```python
from build123d import *

# Parameters (mm, degrees)
F0_R     = 11.2
F0_R_2   = 13.2
F1_DEPTH = 7


with BuildPart() as f1:
    # F0 (on Top) → F1 (new body)
    with BuildSketch(Plane.XY):
        with BuildLine():
            ThreePointArc((6.699736, 20.60143), (11.46029, 25.424858), (13.2, 31.9748))
            ThreePointArc((13.2, 31.9748), (13.048167, 33.971132), (12.59616, 35.921539))
            ThreePointArc((12.59616, 35.921539), (11.664432, 38.15388), (10.34098, 40.17871))
            ThreePointArc((10.34098, 40.17871), (-6.83944, 43.26471), (-12.059859, 26.608256))
            ThreePointArc((-12.059859, 26.608256), (-10.553777, 24.046509), (-8.512807, 21.886583))
            ThreePointArc((-8.512807, 21.886583), (-6.711654, 20.60846), (-4.722613, 19.64853))
            ThreePointArc((-4.722613, 19.64853), (-0.715754, 18.79422), (3.360055, 19.209612))
            ThreePointArc((3.360055, 19.209612), (5.077808, 19.790553), (6.699736, 20.60143))
        make_face()
        with Locations((0, 31.9748)):
            Circle(F0_R, mode=Mode.SUBTRACT)
        with BuildLine():
            ThreePointArc((10.34098, 40.17871), (11.664432, 38.15388), (12.59616, 35.921539))
            ThreePointArc((12.59616, 35.921539), (18.781531, 26.896904), (19.593705, 15.986211))
            ThreePointArc((19.593705, 15.986211), (21.142377, 14.729254), (22.578902, 13.345517))
            ThreePointArc((22.578902, 13.345517), (21.814507, 29.204192), (10.34098, 40.17871))
        make_face()
        with BuildLine():
            ThreePointArc((19.593705, 15.986211), (13.490319, 19.253765), (6.699736, 20.60143))
            ThreePointArc((6.699736, 20.60143), (5.077808, 19.790553), (3.360055, 19.209612))
            ThreePointArc((3.360055, 19.209612), (17.479874, 11.47432), (23.21074, -3.570985))
            ThreePointArc((23.21074, -3.570985), (26.101776, -2.883416), (29.073356, -2.859984))
            ThreePointArc((29.073356, -2.859984), (27.386598, 5.868135), (22.578902, 13.345517))
            ThreePointArc((22.578902, 13.345517), (21.142377, 14.729254), (19.593705, 15.986211))
        make_face()
        with BuildLine():
            ThreePointArc((-8.512807, 21.886583), (-10.553777, 24.046509), (-12.059859, 26.608256))
            ThreePointArc((-12.059859, 26.608256), (-18.775253, 20.783423), (-22.847008, 12.881144))
            ThreePointArc((-22.847008, 12.881144), (-23.327096, 10.945209), (-23.641317, 8.97554))
            ThreePointArc((-23.641317, 8.97554), (-23.419409, 2.056076), (-21.191229, -4.498574))
            ThreePointArc((-21.191229, -4.498574), (-19.678026, -5.497766), (-18.316039, -6.694913))
            ThreePointArc((-18.316039, -6.694913), (-18.67699, 9.400855), (-8.512807, 21.886583))
        make_face()
        with BuildLine():
            ThreePointArc((23.21074, -3.570985), (21.203277, -4.491767), (19.377433, -5.734362))
            ThreePointArc((19.377433, -5.734362), (16.634148, -8.777249), (14.955984, -12.514699))
            ThreePointArc((14.955984, -12.514699), (14.600218, -14.292788), (14.491494, -16.102856))
            ThreePointArc((14.491494, -16.102856), (17.425303, -24.285333), (24.810885, -28.869364))
            ThreePointArc((24.810885, -28.869364), (27.210013, -29.178634), (29.625294, -29.044906))
            ThreePointArc((29.625294, -29.044906), (37.685308, -24.610253), (40.890989, -15.9874))
            ThreePointArc((40.890989, -15.9874), (37.501372, -7.155844), (29.073356, -2.859984))
            ThreePointArc((29.073356, -2.859984), (26.101776, -2.883416), (23.21074, -3.570985))
        make_face()
        with Locations((27.690989, -15.9874)):
            Circle(F0_R, mode=Mode.SUBTRACT)
        with BuildLine():
            ThreePointArc((-23.641317, 8.97554), (-23.327096, 10.945209), (-22.847008, 12.881144))
            ThreePointArc((-22.847008, 12.881144), (-36.198826, 4.289821), (-39.966273, -11.133804))
            ThreePointArc((-39.966273, -11.133804), (-38.874445, -8.975245), (-37.407045, -7.052174))
            ThreePointArc((-37.407045, -7.052174), (-32.684167, 2.816831), (-23.641317, 8.97554))
        make_face()
        with BuildLine():
            ThreePointArc((-14.65482, -13.914168), (-15.918395, -10.016971), (-18.316039, -6.694913))
            ThreePointArc((-18.316039, -6.694913), (-19.678026, -5.497766), (-21.191229, -4.498574))
            ThreePointArc((-21.191229, -4.498574), (-29.744367, -2.948089), (-37.407045, -7.052174))
            ThreePointArc((-37.407045, -7.052174), (-38.874445, -8.975245), (-39.966273, -11.133804))
            ThreePointArc((-39.966273, -11.133804), (-34.048618, -27.555484), (-17.013496, -23.748273))
            ThreePointArc((-17.013496, -23.748273), (-15.547999, -21.163093), (-14.697934, -18.315599))
            ThreePointArc((-14.697934, -18.315599), (-14.542827, -17.156089), (-14.490989, -15.9874))
            ThreePointArc((-14.490989, -15.9874), (-14.53201, -14.947552), (-14.65482, -13.914168))
        make_face()
        with Locations((-27.690989, -15.9874)):
            Circle(F0_R, mode=Mode.SUBTRACT)
        with BuildLine():
            ThreePointArc((14.491494, -16.102856), (14.600218, -14.292788), (14.955984, -12.514699))
            ThreePointArc((14.955984, -12.514699), (1.197116, -20.875175), (-14.697934, -18.315599))
            ThreePointArc((-14.697934, -18.315599), (-15.547999, -21.163093), (-17.013496, -23.748273))
            ThreePointArc((-17.013496, -23.748273), (-8.611345, -26.651557), (0.268106, -26.226661))
            ThreePointArc((0.268106, -26.226661), (2.184719, -25.674462), (4.047613, -24.961751))
            ThreePointArc((4.047613, -24.961751), (9.92909, -21.309841), (14.491494, -16.102856))
        make_face()
        with BuildLine():
            ThreePointArc((0.268106, -26.226661), (14.384319, -33.494013), (29.625294, -29.044906))
            ThreePointArc((29.625294, -29.044906), (27.210013, -29.178634), (24.810885, -28.869364))
            ThreePointArc((24.810885, -28.869364), (13.902636, -29.713735), (4.047613, -24.961751))
            ThreePointArc((4.047613, -24.961751), (2.184719, -25.674462), (0.268106, -26.226661))
        make_face()
        with BuildLine():
            ThreePointArc((19.377433, -5.734362), (15.146889, 9.163701), (3.360055, 19.209612))
            ThreePointArc((3.360055, 19.209612), (-0.715754, 18.79422), (-4.722613, 19.64853))
            ThreePointArc((-4.722613, 19.64853), (-15.509442, 8.535741), (-18.316039, -6.694913))
            ThreePointArc((-18.316039, -6.694913), (-15.918395, -10.016971), (-14.65482, -13.914168))
            ThreePointArc((-14.65482, -13.914168), (0.362553, -17.699441), (14.955984, -12.514699))
            ThreePointArc((14.955984, -12.514699), (16.634148, -8.777249), (19.377433, -5.734362))
        make_face()
        Circle(F0_R_2, mode=Mode.SUBTRACT)
        Circle(F0_R_2)
        Circle(F0_R, mode=Mode.SUBTRACT)
    extrude(amount=F1_DEPTH)


solid = f1.part
```
Part model, mm, in its own coordinate system. A direction names the side the tool comes from. Round coordinates to 2 decimals unless told otherwise and drop trailing zeros. Write each loop counter-clockwise with the first axis right and the second up, starting at its lowest first coordinate (ties: lowest second). Pieces come first, ordered by that corner, then holes. Notation, with made-up numbers: M 1,82 L 12,82 A17 cw 12,102 Z; hole C 14,-24 d11. An arc over 180 degrees is marked long. One line per question, with ' | ' between items.
(1) Probe line 1 along X through (y, z) = (-1, 3.5); line 2 along X through (y, z) = (16.5, 1); line 3 along X through (y, z) = (-9, 2). List the from-to ranges inside material, lowest first.
Answer key:
line 1: x = -38.95 to -35.29, -22.65 to -19.76, -18.35 to -11.16, 11.16 to 19.04, 23.04 to 29 | line 2: x = -21.45 to -14.75, -9.23 to 8.15, 11.29 to 18.87, 19.69 to 23.4 | line 3: x = -40.16 to -36.44, -18.94 to -6.67, 6.67 to 18.94, 36.44 to 38.89
(2) Saw through at C-C on y = 0. Write the cut outline in (x, z), then the cut area to 3 significant figures.
Answer key:
outline: M -38.57,0 L -34.72,0 L -34.72,7 L -38.57,7 Z; M -22.95,0 L -19.86,0 L -19.86,7 L -22.95,7 Z; M -18.22,0 L -11.2,0 L -11.2,7 L -18.22,7 Z; M 11.2,0 L 18.86,0 L 18.86,7 L 11.2,7 Z; M 22.9,0 L 28.9,0 L 28.9,7 L 22.9,7 Z | area: 193 mm^2
(3) Saw through at B-B on z = 1.25. Count the separate pieces of the cut face and the enclosed holes in it, then the cut area to 3 significant figures.
Answer key:
separate pieces: 1 | enclosed holes: 10 | area: 1,900 mm^2
(4) 3-axis set-ups, long thin cutter, end or side, ignore diameter. For faces 4 (the face through (0, 12, 0)), 5 (the face through (-14.544, -17.172, 3.451)): which of +Z, -Z, +X, -X, +Y, -Y reach the whole face in a straight line?
Answer key:
face 4: -Z, +X, -X, +Y, -Y | face 5: +Z, -Z
(5) Pin check, flat tips, straight feed: pin 1 (18 mm diameter, centred on x = 0, y = 31.97, fed in from +Z) (1 decimal); pin 2 (4 mm diameter, centred on x = 32, z = 5.5, fed in from -Y); pin 3 (1 mm diameter, centred on x = 22, z = 2, fed in from +Y). Stop position of each tip, or through.
Answer key:
pin 1: passes through | pin 2: stops at y = -28.98 | pin 3: stops at y = 29.86
(6) Saw through at A-A on x = -6. Write the cut outline in (y, z), then the cut area to 3 significant figures.
Answer key:
outline: M -26.88,0 L -21.15,0 L -21.15,7 L -26.88,7 Z; M -17.24,0 L -9.46,0 L -9.46,7 L -17.24,7 Z; M 9.46,0 L 18.89,0 L 18.89,7 L 9.46,7 Z; M 20.22,0 L 22.52,0 L 22.52,7 L 20.22,7 Z; M 41.43,0 L 43.73,0 L 43.73,7 L 41.43,7 Z | area: 193 mm^2
(7) Two-plate mould, pull along Y, no slides. Class faces 1 (the face through (0.14, -17.71, 3.45)), 2 (the face through (0, 12, 7)), 3 (the face through (-8.735, -26.633, 3.451)): released by +Y, released by -Y, zero draft, split by the parting line, or undercut.
Answer key:
face 1: undercut | face 2: zero draft | face 3: released by -Y
